Could you check a few things on this model? Use its own coordinates, in mm. Give positions to 0.01 mm unless a question says otherwise; leave off trailing zeros. Write each loop counter-clockwise with the first axis right and the second up, starting at its lowest first coordinate (ties: lowest second). Pieces come first, ordered by that corner, then holes. Notation, with made-up numbers: M 39.5,-9.5 L 80.5,-9.5 A12 cw 80.5,13.5 Z; hole C 86,10.5 d9. An arc over 180 degrees is marked long. Use one line per item in the form item = value.
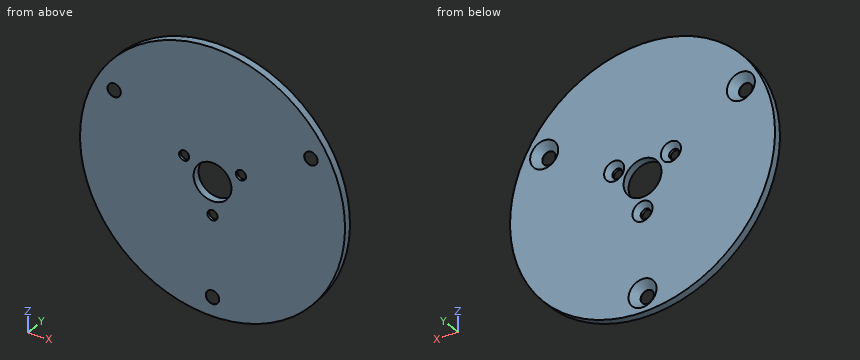
from build123d import *

# Parameters (mm, degrees)
SKETCH1_R                                      = 44.45
BOSS_EXTRUDE1_DEPTH                            = 2.54
CSK_FOR_M4_FLAT_HEAD_MACHINE_SCREW1_AT_2_COUNT = 2
CSK_FOR_M4_FLAT_HEAD_MACHINE_SCREW1_AT_2_PITCH = 65.991135768
CSK_FOR_M4_FLAT_HEAD_MACHINE_SCREW1_AT_3_COUNT = 2
CSK_FOR_M4_FLAT_HEAD_MACHINE_SCREW1_AT_3_PITCH = 65.991135768
SKETCH11_R                                     = 6.35
CUT_EXTRUDE1_DEPTH                             = 63.913087669
CSK_FOR_M3_SFHCS1_AT_2_COUNT                   = 2
CSK_FOR_M3_SFHCS1_AT_2_PITCH                   = 19.052558883
CSK_FOR_M3_SFHCS1_AT_3_COUNT                   = 2
CSK_FOR_M3_SFHCS1_AT_3_PITCH                   = 19.052558883


with BuildPart() as part:
    # Sketch1 → Boss-Extrude1 (new body)
    with BuildSketch(Plane(origin=(0, 0, 0), x_dir=(1, 0, 0), z_dir=(0, 1, 0))):
        with Locations(Location((0, 0, 0), (0, 0, 270))):
            Circle(SKETCH1_R)
    extrude(amount=BOSS_EXTRUDE1_DEPTH)

    # Sketch8 → CSK for M4 Flat Head Machine Screw1 (revolve, cut)
    with BuildSketch(Plane(origin=(0, 2.54, -38.1), x_dir=(0, 0, 1), z_dir=(1, 0, 0))):
        Polygon((0, 0), (0, 2.54), (2.25, 2.54), (2.25, 2.45), (4.7, 0), align=None)
    csk_for_m4_flat_head_machine_screw1 = revolve(axis=Axis((0, 8.89, -38.1), (0, -1, 0)), mode=Mode.SUBTRACT)

    # CSK for M4 Flat Head Machine Screw1 at 2: CSK for M4 Flat Head Machine Screw1 ×2
    with Locations(*[Vector(-0.5000000000000039, 0, 0.8660254037844365) * (i * CSK_FOR_M4_FLAT_HEAD_MACHINE_SCREW1_AT_2_PITCH) for i in range(1, CSK_FOR_M4_FLAT_HEAD_MACHINE_SCREW1_AT_2_COUNT)]):
        add(csk_for_m4_flat_head_machine_screw1, mode=Mode.SUBTRACT)

    # CSK for M4 Flat Head Machine Screw1 at 3: CSK for M4 Flat Head Machine Screw1 ×2
    with Locations(*[Vector(0.4999999999999982, 0, 0.8660254037844397) * (i * CSK_FOR_M4_FLAT_HEAD_MACHINE_SCREW1_AT_3_PITCH) for i in range(1, CSK_FOR_M4_FLAT_HEAD_MACHINE_SCREW1_AT_3_COUNT)]):
        add(csk_for_m4_flat_head_machine_screw1, mode=Mode.SUBTRACT)

    # Sketch11 → Cut-Extrude1 (cut, through all)
    with BuildSketch(Plane(origin=(0, 2.54, 0), x_dir=(1, 0, 0), z_dir=(0, 1, 0))):
        with Locations(Location((0, 0, 0), (0, 0, 270))):
            Circle(SKETCH11_R)
    extrude(amount=-CUT_EXTRUDE1_DEPTH, mode=Mode.SUBTRACT)

    # Sketch13 → CSK for M3 SFHCS1 (revolve, cut)
    with BuildSketch(Plane(origin=(0, 2.54, -11), x_dir=(0, 0, 1), z_dir=(1, 0, 0))):
        Polygon((0, 0), (0, 2.54), (1.7, 2.54), (1.7, 1.66), (3.36, 0), align=None)
    csk_for_m3_sfhcs1 = revolve(axis=Axis((0, 8.89, -11), (0, -1, 0)), mode=Mode.SUBTRACT)

    # CSK for M3 SFHCS1 at 2: CSK for M3 SFHCS1 ×2
    with Locations(*[Vector(-0.5, 0, 0.8660254037844387) * (i * CSK_FOR_M3_SFHCS1_AT_2_PITCH) for i in range(1, CSK_FOR_M3_SFHCS1_AT_2_COUNT)]):
        add(csk_for_m3_sfhcs1, mode=Mode.SUBTRACT)

    # CSK for M3 SFHCS1 at 3: CSK for M3 SFHCS1 ×2
    with Locations(*[Vector(0.5, 0, 0.8660254037844387) * (i * CSK_FOR_M3_SFHCS1_AT_3_PITCH) for i in range(1, CSK_FOR_M3_SFHCS1_AT_3_COUNT)]):
        add(csk_for_m3_sfhcs1, mode=Mode.SUBTRACT)


solid = part.part
1) If I drill on L1, parallel to Z at x = -3, y = 1.45; L2, parallel to X at y = 0.05, z = 19.05; L3, parallel to X at y = 0.5, z = 0, over which ranges is the centre line in solid material (lowest first)?
Checked values:
L1 = -44.35 to -40.11, -36.09 to -5.6, 5.6 to 44.35
L2 = -40.16 to -35.25, -30.75 to 30.75, 35.25 to 40.16
L3 = -44.45 to -6.35, 6.35 to 44.45
2) I want a section at C-C, the plane y = 2.15. Please give me the cut outline in (x, z), plus the area to 3 significant figures.
Checked values:
outline = C 0,0 d88.9; hole C -33,19.05 d8.62; hole C -9.53,5.5 d5.94; hole C 0,0 d12.7; hole C 0,-38.1 d8.62; hole C 0,-11 d5.94; hole C 9.53,5.5 d5.94; hole C 33,19.05 d8.62
area = 5,820 mm2
3) I want a section at B-B, the plane z = 19.05. Please give me the cut outline in (x, y).
Checked values:
outline = M -40.16,0 L -35.25,0 L -35.25,0.09 L -37.7,2.54 L -40.16,2.54 Z; M -30.75,0 L 30.75,0 L 30.75,0.09 L 28.3,2.54 L -28.3,2.54 L -30.75,0.09 Z; M 35.25,0 L 40.16,0 L 40.16,2.54 L 37.7,2.54 L 35.25,0.09 Z
4) For pin 1 Ø2 at (x, z) = (0, -11) entering from +Y; pin 2 Ø5 at (x, z) = (0, -38.1) entering from +Y, each with a flat end and sliding along its axis, tell me the tip position at first contact or that it passes through.
Checked values:
pin_1 = through
pin_2 = 0.34
5) I want a section at A-A, the plane z = 0. Please give me the cut outline in (x, y).
Checked values:
outline = M -44.45,0 L -6.35,0 L -6.35,2.54 L -44.45,2.54 Z; M 6.35,0 L 44.45,0 L 44.45,2.54 L 6.35,2.54 Z
6) I want a section at D-D, the plane z = -38.1. Please give me the cut outline in (x, y).
Checked values:
outline = M -22.9,0 L -2.25,0 L -2.25,0.09 L -4.7,2.54 L -22.9,2.54 Z; M 2.25,0 L 22.9,0 L 22.9,2.54 L 4.7,2.54 L 2.25,0.09 Z
